Autodesk Inventor part; units mm, degrees
ref_plane "YZ Plane" through (0, 0, 0) normal (1, 0, 0) x (0, 1, 0)
ref_plane "XZ Plane" through (0, 0, 0) normal (0, 1, 0) x (-1, 0, 0)
ref_plane "XY Plane" through (0, 0, 0) normal (0, 0, 1) x (1, 0, 0)
sketch "Sketch1" plane through (0, 0, 0) normal (0, 1, 0) x (-1, 0, 0)
  line L0 (0, 0) -> (10, 0)
  line L1 (10, 0) -> (10, -7.5)
  line L2 (10, -7.5) -> (0, -7.5)
  line L3 (0, -7.5) -> (0, 0)
  dimension "d0" = 10
  dimension "d1" = 7.5
extrude "Extrusion1" add sketch "Sketch1" along normal blind 2
sketch "Sketch2" plane through (0, 2, 0) normal (0, 1, 0) x (1, 0, 0)
  line L0 (-10, 7.5) -> (-10, 0)
  line L1 (-10, 0) -> (-5, 0)
  line L2 (-5, 0) -> (-5, 3.75)
  line L3 (-5, 3.75) -> (-10, 3.75)
  line L4 (-10, 3.75) -> (-10, 0)
  circle A0 centre (-5, 3.75) radius 2
  point P0 (0, 0)
  dimension "d4" = 5
  dimension "d5" = 3.75
  dimension "d6" = 4
extrude "Extrusion2" add sketch "Sketch2" along normal blind 7 contours A0 L2 L3 | L3 L2 A0
sketch "Sketch3" plane through (-5, 9, -3.75) normal (0, 1, 0) x (1, 0, 0)
  circle A0 centre (0, 0) radius 1
  point P0 (5, -3.75)
  dimension "d9" = 2
extrude "Extrusion3" add sketch "Sketch3" along normal blind 7
properties part number "LaserMountMount"
Source: CAD feature listing. Evaluate the final solid. Frame: model axes, mm. A direction names the side the tool comes from. Give positions to 0.01 mm unless a question says otherwise; leave off trailing zeros. Order: outer loops, then holes, each group sorted by start corner. A loop starts at its lowest first (then second) coordinate and runs counter-clockwise, first axis right, second up. Notation, with made-up numbers: (7.25, -23) -> (11.25, -23) arc R25 cw to (11.25, -6) -> close; hole circle Ø3 at (14, 0). An arc over 180 degrees is marked (long way). Write item = value, one per line.
Q1. Cut plane B-B, the plane x = -5. Output: boundary loops of the cut face in (y, z).
Data:
outline = (0, -7.5) -> (2, -7.5) -> (2, -5.75) -> (9, -5.75) -> (9, -4.75) -> (16, -4.75) -> (16, -2.75) -> (9, -2.75) -> (9, -1.75) -> (2, -1.75) -> (2, 0) -> (0, 0) -> close
Q2. Pin query (flat end, axial travel): pin 1 (4 mm diameter, centred on x = -7.5, z = -1.5, fed in from -Y); pin 2 (4 mm diameter, centred on y = 5, z = -6, fed in from -X); pin 3 (3 mm diameter, centred on x = -9, z = -5.5, fed in from +Y). Return the tip coordinate at first contact, or that it passes through.
Data:
pin_1 = 0
pin_2 = -6.98
pin_3 = 2
Q3. Cut plane A-A, the plane z = -3.75. Output: boundary loops of the cut face in (x, y).
Data:
outline = (-10, 0) -> (0, 0) -> (0, 2) -> (-3, 2) -> (-3, 9) -> (-4, 9) -> (-4, 16) -> (-6, 16) -> (-6, 9) -> (-7, 9) -> (-7, 2) -> (-10, 2) -> close
Q4. Cut plane D-D, the plane x = -6.25. Output: boundary loops of the cut face in (y, z).
Data:
outline = (0, -7.5) -> (2, -7.5) -> (2, -5.31) -> (9, -5.31) -> (9, -2.19) -> (2, -2.19) -> (2, 0) -> (0, 0) -> close
Q5. Material intervals for line 1 (Y direction, x = -3.5, z = -1.5); line 2 (Y direction, x = -6.75, z = -3.25); line 3 (Z direction, x = -5, y = 15.75), sorted ascending. Write a range as from..to.
Data:
line_1 = 0..2
line_2 = 0..9
line_3 = -4.75..-2.75
Q6. Set-up query: faces 1 (the face through (-5.737, 12.451, -3.074)), 2 (the face through (-5, 1, -7.5)). Return all of +Z, -Z, +X, -X, +Y, -Y with unobstructed straight access to the full face (end or side cutting, diameter ignored); none if empty.
Data:
face_1 = +Y
face_2 = -Z, +X, -X, +Y, -Y
Q7. Cut plane C-C, the plane y = 9.75. Output: boundary loops of the cut face in (x, z).
Data:
outline = circle Ø2 at (-5, -3.75)
